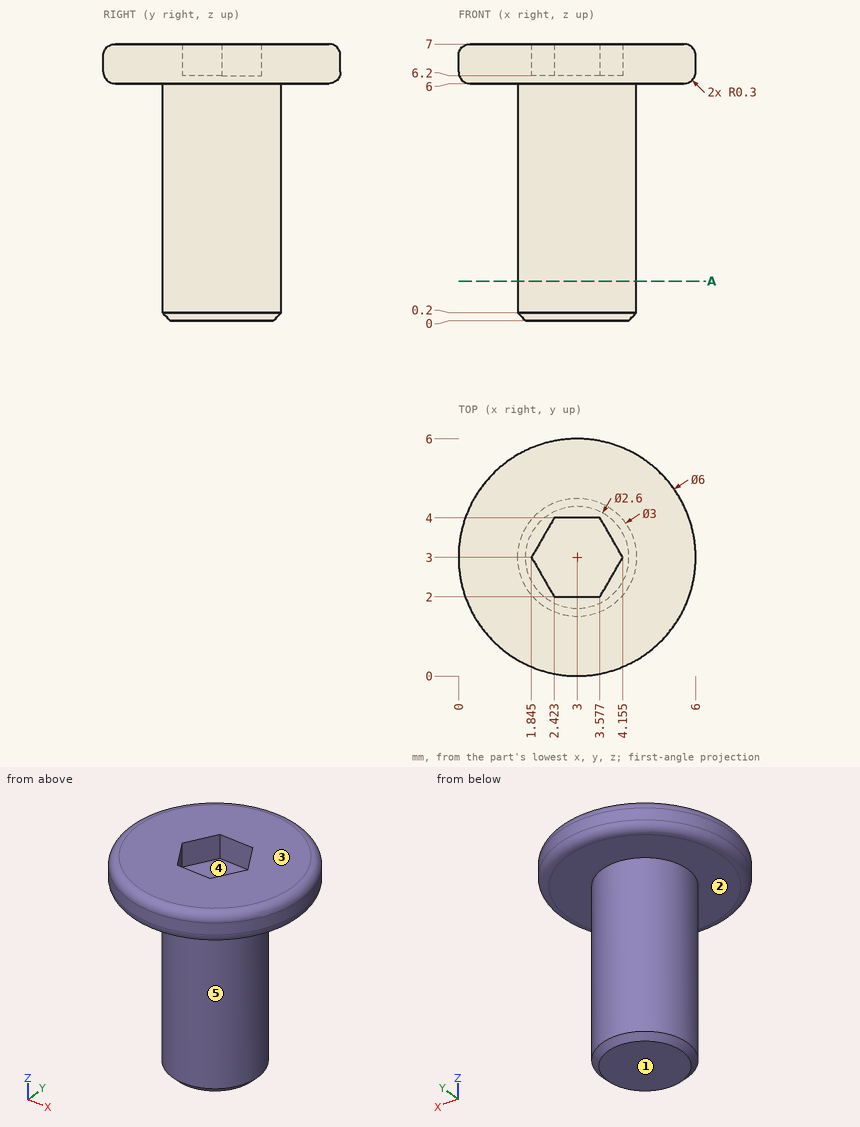
Can you work these out from the drawing? Everything is in mm from the part's minimum corner. A direction names the side the tool comes from. Coordinates: 2 decimals unless noted, no trailing zeros. Loops run counter-clockwise (first coordinate to the right, second up) from the corner with the lowest first, then second, coordinate; pieces in that order, holes last.
1) I need wall thicknesses on probe 1 along Z at (x, y) = (3.5, 1); probe 2 along Y at (x, z) = (3, 5); probe 3 along Z at (x, y) = (2.75, 2.75). Which ranges of each line are inside material? Lowest first, please.
2) Which directions (+Z, -Z, +X, -X, +Y, -Y) give clear straight access to the entire face, cutting with the end or side of a thin tool? Please do the marked faces 1 and 2.
3) Thinking about a two-plate mould opening in Y: for the marked faces 3, 4 and 5, which applies, pulls with the +Y half, pulls with the -Y half, needs draft (parallel to the pull), parting line crosses it, or undercut?
4) Imagine slicing it at A-A on z = 1. List the corners of the cut face in (x, y) for me.
Completed:
1. probe 1: z = 6 to 7
1. probe 2: y = 1.5 to 4.5
1. probe 3: z = 0 to 6.2
2. face 1: -Z, +X, -X, +Y, -Y
2. face 2: -Z
3. face 3: needs draft
3. face 4: undercut
3. face 5: parting line crosses it
4. outline: circle Ø3 at (3, 3)
